Work out the finished part from the listing and answer in its coordinate system (mm). Coordinates: 2 decimals unless noted, no trailing zeros. Write each loop counter-clockwise with the first axis right and the second up, starting at its lowest first coordinate (ties: lowest second). Pieces come first, ordered by that corner, then holes. Notation, with made-up numbers: M -20,44 L -10,44 A23 ccw -10,74 Z; hole C -26.75,6.25 d2. An arc over 180 degrees is marked long. Answer as CSV lines item,"result". Start each with the question number.
(1) A cutting plane is placed at A-A on x = 109.5. Give the vertices of the cut face in (y, z), then the cut area to 3 significant figures.
(2) Flat-ended cylindrical pins translate along their axes: P1, Ø0.8, axis at y = 39.5, z = 2, coming from the -X side; P2, Ø2, axis at y = 39.5, z = 2, coming from the +X side; P3, Ø1.2, axis at x = 146, z = 1.5, coming from the +Y side. Find the tip coordinate at first contact, or state that the pin passes through.
(3) Find the intervals of material crossed by L1, parallel to Y at x = 89.5, z = 3.15, in increasing order. Write a range as [from, to].
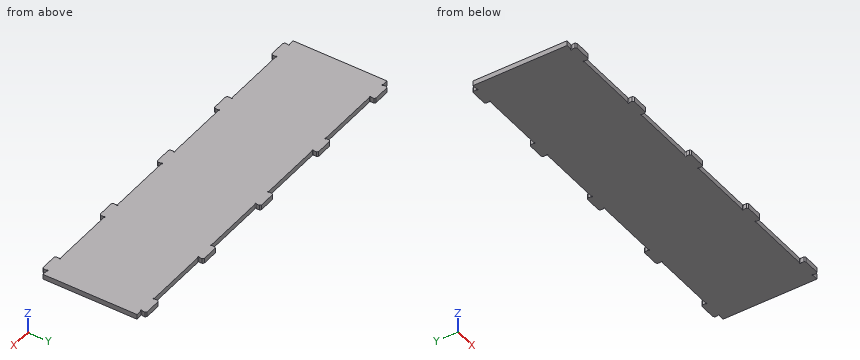
Autodesk Inventor part; units mm, degrees
ref_plane "Plan YZ" through (0, 0, 0) normal (1, 0, 0) x (0, 1, 0)
ref_plane "Plan XZ" through (0, 0, 0) normal (0, 1, 0) x (-1, 0, 0)
ref_plane "Plan XY" through (0, 0, 0) normal (0, 0, 1) x (1, 0, 0)
sketch "Esquisse1" plane through (0, 0, 0) normal (0, 0, 1) x (1, 0, 0)
  line L0 (-142.5, 41.5) -> (-142.5, 37.5)
  line L1 (-142.5, 41.5) -> (-127.5, 41.5)
  line L2 (-127.5, 41.5) -> (-127.5, 37.5)
  line L3 (0, -58.1) -> (0, 58.1) construction
  line L4 (-206.5, 0) -> (206.5, 0) construction
  line L5 (-75, 41.5) -> (-75, 37.5)
  line L6 (-75, 41.5) -> (-60, 41.5)
  line L7 (-60, 41.5) -> (-60, 37.5)
  line L8 (-7.5, 41.5) -> (-7.5, 37.5)
  line L9 (-7.5, 41.5) -> (7.5, 41.5)
  line L10 (7.5, 41.5) -> (7.5, 37.5)
  line L11 (60, 41.5) -> (60, 37.5)
  line L12 (60, 41.5) -> (75, 41.5)
  line L13 (75, 41.5) -> (75, 37.5)
  line L14 (127.5, 41.5) -> (127.5, 37.5)
  line L15 (127.5, 41.5) -> (142.5, 41.5)
  line L16 (142.5, 41.5) -> (142.5, 37.5)
  line L17 (-127.5, 37.5) -> (-75, 37.5)
  line L18 (-60, 37.5) -> (-7.5, 37.5)
  line L19 (7.5, 37.5) -> (60, 37.5)
  line L20 (75, 37.5) -> (127.5, 37.5)
  line L21 (142.5, 37.5) -> (147.5, 37.5)
  line L22 (-142.5, 37.5) -> (-147.5, 37.5)
  line L23 (-142.5, -41.5) -> (-142.5, -37.5)
  line L24 (-142.5, -41.5) -> (-127.5, -41.5)
  line L25 (-127.5, -41.5) -> (-127.5, -37.5)
  line L26 (-75, -41.5) -> (-75, -37.5)
  line L27 (-75, -41.5) -> (-60, -41.5)
  line L28 (-60, -41.5) -> (-60, -37.5)
  line L29 (-7.5, -41.5) -> (-7.5, -37.5)
  line L30 (-7.5, -41.5) -> (7.5, -41.5)
  line L31 (7.5, -41.5) -> (7.5, -37.5)
  line L32 (60, -41.5) -> (60, -37.5)
  line L33 (60, -41.5) -> (75, -41.5)
  line L34 (75, -41.5) -> (75, -37.5)
  line L35 (127.5, -41.5) -> (127.5, -37.5)
  line L36 (127.5, -41.5) -> (142.5, -41.5)
  line L37 (142.5, -41.5) -> (142.5, -37.5)
  line L38 (-127.5, -37.5) -> (-75, -37.5)
  line L39 (-60, -37.5) -> (-7.5, -37.5)
  line L40 (7.5, -37.5) -> (60, -37.5)
  line L41 (75, -37.5) -> (127.5, -37.5)
  line L42 (142.5, -37.5) -> (147.5, -37.5)
  line L43 (-142.5, -37.5) -> (-147.5, -37.5)
  line L44 (147.5, -37.5) -> (147.5, 37.5)
  line L45 (-147.5, -37.5) -> (-147.5, 37.5)
  point P0 (0, 0)
  dimension "d1" = 15
  dimension "d3" = 4
  dimension "d6" = 67.5
  dimension "d11" = 5
  dimension "d12" = 5
  dimension "d30" = 75
extrude "Extrusion1" add sketch "Esquisse1" along normal blind 4
sketch "Esquisse6" plane through (0, 0, 4) normal (0, 0, 1) x (1, 0, 0)
  line L0 (0, -58.1) -> (0, 58.1) construction
  line L1 (-206.5, 0) -> (206.5, 0) construction
  point P0 (0, 0)
  point P1 (-142.5, 37.5)
  point P2 (-127.5, 37.5)
  point P3 (-75, 37.5)
  point P4 (-60, 37.5)
  point P5 (-7.5, 37.5)
  point P6 (7.5, 37.5)
  point P7 (60, 37.5)
  point P8 (75, 37.5)
  point P9 (142.5, 37.5)
  point P10 (127.5, 37.5)
  point P11 (-142.5, -37.5)
  point P12 (-127.5, -37.5)
  point P13 (-75, -37.5)
  point P14 (-60, -37.5)
  point P15 (-7.5, -37.5)
  point P16 (7.5, -37.5)
  point P17 (60, -37.5)
  point P18 (75, -37.5)
  point P19 (142.5, -37.5)
  point P20 (127.5, -37.5)
hole "Perçage1" at (-142.5, 37.5, 4) at (-127.5, 37.5, 4) at (-75, 37.5, 4) at (-60, 37.5, 4) at (-7.5, 37.5, 4) at (7.5, 37.5, 4) at (60, 37.5, 4) at (75, 37.5, 4) at (142.5, 37.5, 4) at (127.5, 37.5, 4) at (127.5, -37.5, 4) at (142.5, -37.5, 4) at (75, -37.5, 4) at (60, -37.5, 4) at (7.5, -37.5, 4) at (-7.5, -37.5, 4) at (-60, -37.5, 4) at (-75, -37.5, 4) at (-127.5, -37.5, 4) at (-142.5, -37.5, 4) direction (0, 0, -1) diameter 1 end through all
chamfer "Chanfrein1" distance 1 angle 45 20 edges at (-142.5, 41.5, 2) (-127.5, 41.5, 2) (-75, 41.5, 2) (-60, 41.5, 2) (-7.5, 41.5, 2) (7.5, 41.5, 2) (60, 41.5, 2) (75, 41.5, 2) (127.5, 41.5, 2) (142.5, 41.5, 2) (142.5, -41.5, 2) (127.5, -41.5, 2) (60, -41.5, 2) (75, -41.5, 2) (-142.5, -41.5, 2) (-127.5, -41.5, 2) (-75, -41.5, 2) (-60, -41.5, 2) (-7.5, -41.5, 2) (7.5, -41.5, 2)
properties part number "P1704_003" material "Plastique PMMA"
Here are the results:
1,outline,"M -37.5,0 L 37.5,0 L 37.5,4 L -37.5,4 Z"
1,area,"300 mm^2"
2,P1,"stops at x = -142.5"
2,P2,"stops at x = 142.5"
2,P3,"stops at y = 37.5"
3,L1,"y = [-37.5, 37.5]"
